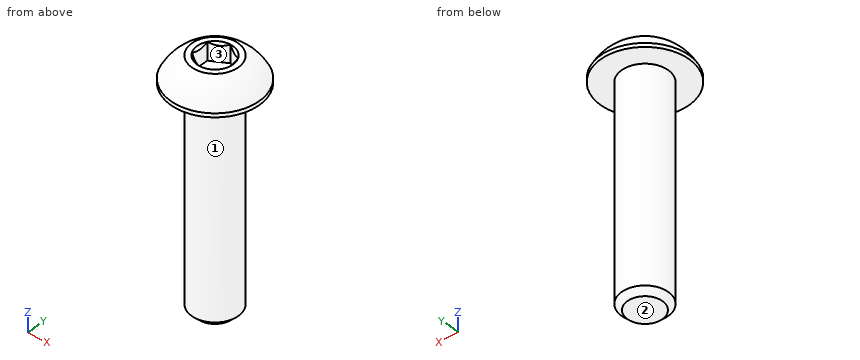
```python
from build123d import *

# Parameters (mm, degrees)
CUT_EXTRUDE2_DEPTH = 1.155


with BuildPart() as part:
    # Sketch10 → Revolve3 (revolve)
    with BuildSketch(Plane(origin=(0, 0, 0), x_dir=(0, 0, -1), z_dir=(1, 0, 0)), mode=Mode.PRIVATE) as revolve3_sk:
        Polygon((15.275, 1.5), (15.65, 1.125), (15.65, 0), (1.65, 0), (1.65, 1.5), align=None)
    revolve(revolve3_sk.sketch.rotate(Axis((0, 0, 0), (0, 0, -1)), 90), axis=Axis((0, 0, 0), (0, 0, -1)))

    # Sketch7 → Revolve2 (revolve)
    with BuildSketch(Plane(origin=(0, 0, 0), x_dir=(0, 0, -1), z_dir=(1, 0, 0)), mode=Mode.PRIVATE) as revolve2_sk:
        with BuildLine():
            Line((1.4025, 2.85), (1.65, 2.85))
            Line((1.65, 2.85), (1.65, 0))
            Line((1.65, 0), (0, 0))
            Line((0, 0), (0, 1.5))
            ThreePointArc((0, 1.5), (0.59512511, 2.285251969), (1.4025, 2.85))
        make_face()
    revolve(revolve2_sk.sketch.rotate(Axis((0, 0, 0), (0, 0, -1)), 180), axis=Axis((0, 0, 0), (0, 0, -1)))

    # Sketch5 → Cut-Extrude2 (cut)
    with BuildSketch(Plane.XY):
        Polygon((1, -0.577350269), (1, 0.577350269), (0, 1.154700538), (-1, 0.577350269), (-1, -0.577350269), (0, -1.154700538), align=None)
    extrude(amount=-CUT_EXTRUDE2_DEPTH, mode=Mode.SUBTRACT)

    # Cut-Extrude3 cone 1 section (on through the dimple's axis) → Cut-Extrude3 (revolve, cut)
    with BuildSketch(Plane(origin=(0, 0, 0), x_dir=(0, -1, 0), z_dir=(1, 0, 0))):
        Polygon((0, 0), (1.154700538, 0), (0, 1.154700538), align=None)
    revolve(axis=Axis((0, 0, 0), (0, 0, -1)), mode=Mode.SUBTRACT)


solid = part.part
```
Can you work these out from the model? Positions are in its coordinate system, mm. Face numbers are marked on the shaded views. Coordinates: 2 decimals unless noted, no trailing zeros. Loops run counter-clockwise (first coordinate to the right, second up) from the corner with the lowest first, then second, coordinate; pieces in that order, holes last.
1) Imagine slicing it at C-C on x = 2. List the corners of the cut face in (y, z) for me, plus the area to 3 significant figures.
2) For pin 1 (0.9 mm diameter, centred on y = 0, z = -0.5, fed in from -X); pin 2 (2 mm diameter, centred on y = 0, z = -10, fed in from +X); pin 3 (1.3 mm diameter, centred on y = 0, z = -0.5, fed in from +X), each with a flat end and sliding along its axis, tell me the tip position at first contact or that it passes through.
3) Thinking about a two-plate mould opening in Y: for the marked faces 1, 2 and 3, which applies, pulls with the +Y half, pulls with the -Y half, needs draft (parallel to the pull), parting line crosses it, or undercut?
4) I need wall thicknesses on probe 1 along Z at (x, y) = (0.6, -0.7) (3 decimals); probe 2 along X at (y, z) = (0.05, -11.5); probe 3 along X at (y, z) = (0.4, -11.75). Which ranges of each line are inside material? Lowest first, please.
5) Imagine slicing it at B-B on z = -14. List the corners of the cut face in (x, y) for me.
6) Imagine slicing it at D-D on y = 1.95. List the corners of the cut face in (x, z) for me, plus the area to 3 significant figures.
Completed:
1. outline: (-2.03, -1.65) - (2.03, -1.65) - (2.03, -1.4) arc R2.46 ccw to (-2.03, -1.4) - close
1. area: 4.06 mm2
2. pin 1: stops at x = -2.58
2. pin 2: stops at x = 1.5
2. pin 3: stops at x = 2.71
3. face 1: parting line crosses it
3. face 2: needs draft
3. face 3: undercut
4. probe 1: z = -15.65 to -1.155
4. probe 2: x = -1.5 to 1.5
4. probe 3: x = -1.45 to 1.45
5. outline: circle Ø3 at (0, 0)
6. outline: (-2.08, -1.65) - (2.08, -1.65) - (2.08, -1.4) arc R2.5 ccw to (-2.08, -1.4) - close
6. area: 4.27 mm2
